from build123d import *

# Parameters (mm, degrees)
F0_R     = 5.08
F1_DEPTH = 5.08
F2_SIZE  = 5.07999


# Not quite as in the source:
# - a fillet or chamfer is up to 0.001 mm smaller than in the source, because OpenCascade refuses the exact size


with BuildPart() as f1:
    # F0 (on Top) → F1 (new body)
    with BuildSketch(Plane.XY):
        with BuildLine():
            ThreePointArc((-16.3226491362, 0), (-11.5418558911, 11.5418558911), (0, 16.3226491362))
            Line((0, 16.3226491362), (-30.0371784096, 30.0371784096))
            Line((-30.0371784096, 30.0371784096), (-16.3226491362, 0))
        make_face()
        with BuildLine():
            ThreePointArc((0, 16.3226491362), (11.5418558911, 11.5418558911), (16.3226491362, 0))
            Line((16.3226491362, 0), (30.0371784096, 30.0371784096))
            Line((30.0371784096, 30.0371784096), (0, 16.3226491362))
        make_face()
        with BuildLine():
            Line((30.0371784096, -30.0371784096), (16.3226491362, 0))
            ThreePointArc((16.3226491362, 0), (11.5418558911, -11.5418558911), (0, -16.3226491362))
            Line((0, -16.3226491362), (30.0371784096, -30.0371784096))
        make_face()
        with BuildLine():
            Line((-30.0371784096, -30.0371784096), (0, -16.3226491362))
            ThreePointArc((0, -16.3226491362), (-11.5418558911, -11.5418558911), (-16.3226491362, 0))
            Line((-16.3226491362, 0), (-30.0371784096, -30.0371784096))
        make_face()
        with BuildLine():
            ThreePointArc((0, -16.3226491362), (11.5418558911, -11.5418558911), (16.3226491362, 0))
            ThreePointArc((16.3226491362, 0), (11.5418558911, 11.5418558911), (0, 16.3226491362))
            ThreePointArc((0, 16.3226491362), (-11.5418558911, 11.5418558911), (-16.3226491362, 0))
            ThreePointArc((-16.3226491362, 0), (-11.5418558911, -11.5418558911), (0, -16.3226491362))
        make_face()
        Circle(F0_R, mode=Mode.SUBTRACT)
    extrude(amount=F1_DEPTH)

    # F2 (size 5.08 in the source; OpenCascade refuses exactly that, so slightly less here)
    f2_edges = [f1.edges().sort_by_distance(p)[0] for p in [
        (-15.018589, -23.179914, 5.08),
        (-23.179914, -15.018589, 5.08),
        (15.018589, -23.179914, 5.08),
        (23.179914, -15.018589, 5.08),
        (23.179914, 15.018589, 5.08),
        (15.018589, 23.179914, 5.08),
        (-15.018589, 23.179914, 5.08),
        (-23.179914, 15.018589, 5.08),
    ]]
    chamfer(f2_edges, length=F2_SIZE)


solid = f1.part
Design review of the part built by this model. Coordinates are the model's own, in mm. A direction names the side the tool comes from. Coordinates: 2 decimals unless noted, no trailing zeros. Order: outer loops, then holes, each group sorted by start corner. A loop starts at its lowest first (then second) coordinate and runs counter-clockwise, first axis right, second up. Notation, with made-up numbers: M 84.5,63 L 95.5,63 A20 ccw 95.5,74 Z; hole C 50,4 d3. An arc over 180 degrees is marked long. Use a Markdown table: item, result.
(1) For faces 4 (the flat face through (11.24, -18.62, 2.58)), 5 (the flat face through (11.686, 18.827, 2.576)), 6 (the flat face through (18.827, -11.686, 2.576)), 7 (the flat face through (-18.62, -11.24, 2.58)), list the 3-axis set-ups (+Z, -Z, +X, -X, +Y, -Y) from which the entire face can be reached by the end or side of a thin tool; tool diameter is ignored.
Worked answers:
| item | result |
|---|---|
| face 4 | +Z, -Y |
| face 5 | +Z, +Y |
| face 6 | +Z, +X |
| face 7 | +Z, -X |
(2) Draft analysis for pull direction Y (two halves, no side actions). For faces 1 (the flat face through (-11.24, 18.62, 2.58)), 2 (the flat face through (-18.827, 11.686, 2.576)), 3 (the flat face through (-5, 5, 5.08)), state which applies: released by +Y, released by -Y, zero draft, split by the parting line, or undercut.
Worked answers:
| item | result |
|---|---|
| face 1 | released by +Y |
| face 2 | undercut |
| face 3 | zero draft |
(3) Wall thickness on probe 1 along Y at (x, z) = (14.5, 1.9); probe 2 along X at (y, z) = (3, 3.45); probe 3 along X at (y, z) = (21, 1.65): over which ranges is each line inside the solid? List them lowest first.
Worked answers:
| item | result |
|---|---|
| probe 1 | y = -20.85 to -0.58, 0.58 to 20.85 |
| probe 2 | x = -13.9 to -4.1, 4.1 to 13.9 |
| probe 3 | x = -24.1 to -14.22, 14.22 to 24.1 |
(4) For P1, Ø3, axis at x = 5.5, z = 3, coming from the -Y side; P2, Ø1.5, axis at x = 18.5, y = 14, coming from the +Z side, all flat-tipped, find the tip position at first contact; note any pin that passes through.
Worked answers:
| item | result |
|---|---|
| P1 | stops at y = -17.32 |
| P2 | stops at z = 4.58 |
(5) Add section B-B (z = 2.6). Give the boundary of the cut face in (x, y).
Worked answers:
| item | result |
|---|---|
| outline | M -24.78,-24.78 L 0,-13.46 L 24.78,-24.78 L 13.46,0 L 24.78,24.78 L 0,13.46 L -24.78,24.78 L -13.46,0 Z; hole C 0,0 d10.16 |
